Part model, mm, in its own coordinate system. Coordinates: 2 decimals unless noted, no trailing zeros. Use one line per item in the form item = value. Start each with the question number.
(1) Pin check, flat tips, straight feed: P1, Ø3, axis at y = 288, z = 0.5, coming from the +X side; P2, Ø12, axis at x = 62.5, y = 198, coming from the -Z side; P3, Ø16, axis at x = -0.63, y = 25, coming from the +Z side; P4, Ø2, axis at y = 286, z = -1.5, coming from the +X side. Stop position of each tip, or through.
(2) Mould opens along X. For faces 1 (the cylindrical face through (84.75, 317.59, -0.09)), 2 (the cylindrical face through (51.58, 233.22, -6.21)), 3 (the flat face through (125.33, 460.98, 0.08)) say: +X half, -X half, draft (parallel to the pull), parting line (faces both ways), or undercut.
(3) Band-saw the part on A-A on z = 2.75. Count the separate pieces of the cut face and the enclosed holes in it, then the cut area to 3 significant figures.
(4) Drill centre lines: L1, parallel to X at y = 432.5, z = -1.25; L2, parallel to X at y = 205.5, z = 2.25; L3, parallel to X at y = 83.5, z = 5.25. Where is each one in solid material? Low to high. Write a range as [from, to].
```python
from build123d import *

# Parameters (mm, degrees)
BOSS_EXTRUDE1_DEPTH     = 6.5
CUT_EXTRUDE1_DEPTH      = 493.386170136
CUT_EXTRUDE1_DEPTH_BACK = 493.386170136
SKETCH2_R               = 5
FILLET1_R               = 1


with BuildPart() as part:
    # Sketch1 → Boss-Extrude1 (new, symmetric)
    with BuildSketch(Plane.XY):
        Polygon((0, 0), (129.035423591, 450), (120.599566698, 475), (-15.604491538, 0), align=None)
    extrude(amount=BOSS_EXTRUDE1_DEPTH, both=True)

    # Sketch2 → Cut-Extrude1 (cut, two sides: drawn at the far end of the back side and taken through both)
    with BuildSketch(Plane.XY.offset(6.5).offset(-CUT_EXTRUDE1_DEPTH_BACK)):
        with Locations((-0.633611125, 25)):
            Circle(SKETCH2_R)
        with Locations((15.904630224, 82.675701756)):
            Circle(SKETCH2_R)
        with Locations((32.442871573, 140.351403513)):
            Circle(SKETCH2_R)
        with Locations((48.981112922, 198.027105269)):
            Circle(SKETCH2_R)
        with Locations((65.519354271, 255.702807025)):
            Circle(SKETCH2_R)
        with Locations((82.05759562, 313.378508781)):
            Circle(SKETCH2_R)
        with Locations((98.595836969, 371.054210538)):
            Circle(SKETCH2_R)
        with Locations((115.134078318, 428.729912294)):
            Circle(SKETCH2_R)
    extrude(amount=CUT_EXTRUDE1_DEPTH + CUT_EXTRUDE1_DEPTH_BACK, mode=Mode.SUBTRACT)

    # Fillet1
    fillet1_edges = [part.edges().sort_by_distance(p)[0] for p in [
        (124.817495144, 462.5, 6.5),
        (52.49753758, 237.5, 6.5),
        (-7.802245769, 0, 6.5),
        (52.49753758, 237.5, -6.5),
        (124.817495144, 462.5, -6.5),
        (64.517711796, 225, -6.5),
        (-7.802245769, 0, -6.5),
        (-15.604491538, 0, 0),
        (120.599566698, 475, 0),
        (129.035423591, 450, 0),
        (0, 0, 0),
        (64.517711796, 225, 6.5),
    ]]
    fillet(fillet1_edges, radius=FILLET1_R)


solid = part.part
```
A:
q1.P1 = 83.01
q1.P2 = -6.36
q1.P3 = 6.5
q1.P4 = 82.3
q2.face_1 = undercut
q2.face_2 = -X half
q2.face_3 = +X half
q3.separate_pieces = 1
q3.enclosed_holes = 8
q3.area = 6,590 mm²
q4.L1 = [108.41, 111.85], [118.42, 124.02]
q4.L2 = [43.32, 58.93]
q4.L3 = [8.34, 10.97], [20.84, 23.94]
